Geometry: final body of the model. Coordinates: model frame, mm. Coordinates: 2 decimals unless noted, no trailing zeros. Write each loop counter-clockwise with the first axis right and the second up, starting at its lowest first coordinate (ties: lowest second). Pieces come first, ordered by that corner, then holes. Notation, with made-up numbers: (53, 50) - (106, 50) arc R28 ccw to (106, 70) - close; hole circle Ø2 at (41.5, 49.25). An arc over 180 degrees is marked (long way). Put each result on its own line as item: value.
```python
from build123d import *

# Parameters (mm, degrees)
EXTRUDE_1_DEPTH = 5


with BuildPart() as part:
    # 草圖1 → 填料-伸長1 (new body)
    with BuildSketch(Plane(origin=(0, 0, 0), x_dir=(1, 0, 0), z_dir=(0, 1, 0))):
        with BuildLine():
            Line((27.133974596, -175.834936491), (47, -141.425971147))
            Line((47, -141.425971147), (193.042249331, 111.526624746))
            Line((193.042249331, 111.526624746), (212.908274735, 145.93559009))
            ThreePointArc((212.908274735, 145.93559009), (213.067193357, 146.142696871), (213.274300139, 146.301615494))
            Line((213.274300139, 146.301615494), (223.434554176, 152.167640898))
            ThreePointArc((223.434554176, 152.167640898), (223.900480003, 152.774847256), (223.80057958, 153.533666301))
            Line((223.80057958, 153.533666301), (218.80057958, 162.193920339))
            ThreePointArc((218.80057958, 162.193920339), (218.700679158, 162.952739384), (219.166604984, 163.559945743))
            Line((219.166604984, 163.559945743), (226.094808214, 167.559945743))
            ThreePointArc((226.094808214, 167.559945743), (226.560734041, 168.167152102), (226.460833618, 168.925971147))
            Line((226.460833618, 168.925971147), (212.460833618, 193.174682453))
            ThreePointArc((212.460833618, 193.174682453), (211.853627259, 193.640608279), (211.094808214, 193.540707856))
            Line((211.094808214, 193.540707856), (204.166604984, 189.540707856))
            ThreePointArc((204.166604984, 189.540707856), (203.407785939, 189.440807434), (202.80057958, 189.90673326))
            Line((202.80057958, 189.90673326), (197.80057958, 198.566987298))
            ThreePointArc((197.80057958, 198.566987298), (197.193373221, 199.032913124), (196.434554176, 198.933012702))
            Line((196.434554176, 198.933012702), (186.274300139, 193.066987298))
            ThreePointArc((186.274300139, 193.066987298), (186.033119184, 192.967086876), (185.774300139, 192.933012702))
            Line((185.774300139, 192.933012702), (146.042249331, 192.933012702))
            Line((146.042249331, 192.933012702), (-146.042249331, 192.933012702))
            Line((-146.042249331, 192.933012702), (-185.774300139, 192.933012702))
            ThreePointArc((-185.774300139, 192.933012702), (-186.033119184, 192.967086876), (-186.274300139, 193.066987298))
            Line((-186.274300139, 193.066987298), (-196.434554176, 198.933012702))
            ThreePointArc((-196.434554176, 198.933012702), (-197.193373221, 199.032913124), (-197.80057958, 198.566987298))
            Line((-197.80057958, 198.566987298), (-202.80057958, 189.90673326))
            ThreePointArc((-202.80057958, 189.90673326), (-203.407785939, 189.440807434), (-204.166604984, 189.540707856))
            Line((-204.166604984, 189.540707856), (-211.094808214, 193.540707856))
            ThreePointArc((-211.094808214, 193.540707856), (-211.853627259, 193.640608279), (-212.460833618, 193.174682453))
            Line((-212.460833618, 193.174682453), (-226.460833618, 168.925971147))
            ThreePointArc((-226.460833618, 168.925971147), (-226.560734041, 168.167152102), (-226.094808214, 167.559945743))
            Line((-226.094808214, 167.559945743), (-219.166604984, 163.559945743))
            ThreePointArc((-219.166604984, 163.559945743), (-218.700679158, 162.952739384), (-218.80057958, 162.193920339))
            Line((-218.80057958, 162.193920339), (-223.80057958, 153.533666301))
            ThreePointArc((-223.80057958, 153.533666301), (-223.900480003, 152.774847256), (-223.434554176, 152.167640898))
            Line((-223.434554176, 152.167640898), (-213.274300139, 146.301615494))
            ThreePointArc((-213.274300139, 146.301615494), (-213.067193357, 146.142696871), (-212.908274735, 145.93559009))
            Line((-212.908274735, 145.93559009), (-193.042249331, 111.526624746))
            Line((-193.042249331, 111.526624746), (-47, -141.425971147))
            Line((-47, -141.425971147), (-27.133974596, -175.834936491))
            ThreePointArc((-27.133974596, -175.834936491), (-27.034074174, -176.076117445), (-27, -176.334936491))
            Line((-27, -176.334936491), (-27, -188.066987298))
            ThreePointArc((-27, -188.066987298), (-26.707106781, -188.774094079), (-26, -189.066987298))
            Line((-26, -189.066987298), (-16, -189.066987298))
            ThreePointArc((-16, -189.066987298), (-15.292893219, -189.359880517), (-15, -190.066987298))
            Line((-15, -190.066987298), (-15, -198.066987298))
            ThreePointArc((-15, -198.066987298), (-14.707106781, -198.774094079), (-14, -199.066987298))
            Line((-14, -199.066987298), (14, -199.066987298))
            ThreePointArc((14, -199.066987298), (14.707106781, -198.774094079), (15, -198.066987298))
            Line((15, -198.066987298), (15, -190.066987298))
            ThreePointArc((15, -190.066987298), (15.292893219, -189.359880517), (16, -189.066987298))
            Line((16, -189.066987298), (26, -189.066987298))
            ThreePointArc((26, -189.066987298), (26.707106781, -188.774094079), (27, -188.066987298))
            Line((27, -188.066987298), (27, -176.334936491))
            ThreePointArc((27, -176.334936491), (27.034074174, -176.076117445), (27.133974596, -175.834936491))
        make_face()
    extrude(amount=EXTRUDE_1_DEPTH)


solid = part.part
```
1. Section query B-B (z = -65.5). Return loops of the section in (x, y).
Answer below:
outline: (-166.47, 0) - (166.47, 0) - (166.47, 5) - (-166.47, 5) - close
2. Pin query (flat end, axial travel): pin 1 Ø1.5 at (y, z) = (3.5, 193.5) entering from +X; pin 2 Ø2.5 at (x, y) = (23.5, 3.5) entering from +Z; pin 3 Ø2 at (x, y) = (41, 2.5) entering from -Z. Return the tip coordinate at first contact, or that it passes through.
Answer below:
pin 1: stops at x = 15
pin 2: stops at z = 189.07
pin 3: stops at z = -192.93
3. Section query A-A (x = -1). Return loops of the section in (y, z).
Answer below:
outline: (0, -192.93) - (5, -192.93) - (5, 199.07) - (0, 199.07) - close
4. Ray query, probe 1 along Z at (x, y) = (22.5, 2.35); probe 2 along X at (y, z) = (2.25, 145); probe 3 along Z at (x, y) = (151, 0.7). Return the intervals inside material, ascending. Write a range as from..to.
Answer below:
probe 1: z = -192.93..189.07
probe 2: x = -44.94..44.94
probe 3: z = -192.93..-38.71
